Verification items for the finished model (mm, model axes). Round coordinates to 2 decimals unless told otherwise and drop trailing zeros. Write each loop counter-clockwise with the first axis right and the second up, starting at its lowest first coordinate (ties: lowest second). Pieces come first, ordered by that corner, then holes.
from build123d import *

# Parameters (mm, degrees)
SKETCH1_W           = 114.02881
SKETCH1_H           = 34
BOSS_EXTRUDE1_DEPTH = 10.01
SKETCH8_R           = 2.6
CUT_EXTRUDE3_DEPTH  = 120.410090068
SKETCH11_R          = 1.59
CUT_EXTRUDE6_DEPTH  = 120.410090068
SKETCH12_W          = 34
SKETCH12_H          = 10.01
BOSS_EXTRUDE2_DEPTH = 2.69
SKETCH14_W          = 34
SKETCH14_H          = 10.01
CUT_EXTRUDE7_DEPTH  = 2.69


with BuildPart() as part:
    # Sketch1 → Boss-Extrude1 (new body)
    with BuildSketch(Plane(origin=(0, 0, 0), x_dir=(1, 0, 0), z_dir=(0, 1, 0))):
        with Locations((57.014405, 17)):
            Rectangle(SKETCH1_W, SKETCH1_H)
    extrude(amount=BOSS_EXTRUDE1_DEPTH)

    # Sketch8 → Cut-Extrude3 (cut, through all)
    with BuildSketch(Plane(origin=(0, 0, -34), x_dir=(-1, 0, 0), z_dir=(0, 0, -1))):
        with Locations((-89.8, 5)):
            Circle(SKETCH8_R)
        with Locations((-29.8, 5)):
            Circle(SKETCH8_R)
    extrude(amount=-CUT_EXTRUDE3_DEPTH, mode=Mode.SUBTRACT)

    # Sketch11 → Cut-Extrude6 (cut, through all)
    with BuildSketch(Plane(origin=(0, 10.01, 0), x_dir=(1, 0, 0), z_dir=(0, 1, 0))):
        with Locations(Location((110.52881, 10.5, 0), (0, 0, 270))):
            Circle(SKETCH11_R)
        with Locations(Location((110.52881, 23.5, 0), (0, 0, 270))):
            Circle(SKETCH11_R)
        with Locations(Location((100.52881, 10.5, 0), (0, 0, 270))):
            Circle(SKETCH11_R)
        with Locations(Location((100.52881, 23.5, 0), (0, 0, 270))):
            Circle(SKETCH11_R)
    extrude(amount=-CUT_EXTRUDE6_DEPTH, mode=Mode.SUBTRACT)

    # Sketch12 → Boss-Extrude2 (add)
    with BuildSketch(Plane(origin=(114.02881, 0, 0), x_dir=(0, 0, -1), z_dir=(1, 0, 0))):
        with Locations((17, 5.005)):
            Rectangle(SKETCH12_W, SKETCH12_H)
    extrude(amount=BOSS_EXTRUDE2_DEPTH)

    # Sketch14 → Cut-Extrude7 (cut)
    with BuildSketch(Plane.ZY):
        with Locations((-17, 5.005)):
            Rectangle(SKETCH14_W, SKETCH14_H)
    extrude(amount=-CUT_EXTRUDE7_DEPTH, mode=Mode.SUBTRACT)


solid = part.part
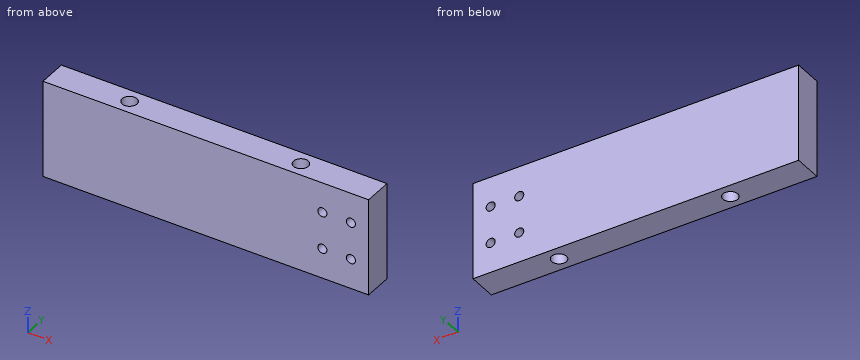
Q1. Material ranges on line 1 along X through (y, z) = (7.75, -11); line 2 along X through (y, z) = (4.25, -30); line 3 along X through (y, z) = (6.5, -23.5), recorded low to high.
Recorded:
line 1: x = 2.69 to 99.02, 102.04 to 109.02, 112.04 to 116.72
line 2: x = 2.69 to 27.31, 32.29 to 87.31, 92.29 to 116.72
line 3: x = 2.69 to 27.68, 31.92 to 87.68, 91.92 to 98.94, 102.12 to 108.94, 112.12 to 116.72
Q2. Sectioned sample at C-C (y = 5). Enter the section's corners in (x, z), plus the area to 3 significant figures.
Recorded:
outline: (2.69, -34) - (27.2, -34) - (27.2, 0) - (2.69, 0) - close; (32.4, -34) - (87.2, -34) - (87.2, 0) - (32.4, 0) - close; (92.4, -34) - (116.72, -34) - (116.72, 0) - (92.4, 0) - close; hole circle Ø3.18 at (100.53, -23.5); hole circle Ø3.18 at (100.53, -10.5); hole circle Ø3.18 at (110.53, -23.5); hole circle Ø3.18 at (110.53, -10.5)
area: 3,490 mm2
Q3. Depth check by flat-ended pin: P1, Ø4, axis at x = 89.8, y = 5, coming from the -Z side; P2, Ø6, axis at x = 38, y = 1, coming from the +Z side. Enter the tip coordinate at first touch or a pass-through.
Recorded:
P1: passes through
P2: stops at z = 0
Q4. Sectioned sample at A-A (z = -10.5). Enter the section's corners in (x, y), plus the area to 3 significant figures.
Recorded:
outline: (2.69, 0) - (98.94, 0) - (98.94, 10.01) - (2.69, 10.01) - close; (102.12, 0) - (108.94, 0) - (108.94, 10.01) - (102.12, 10.01) - close; (112.12, 0) - (116.72, 0) - (116.72, 10.01) - (112.12, 10.01) - close; hole circle Ø5.2 at (29.8, 5); hole circle Ø5.2 at (89.8, 5)
area: 1,040 mm2
Q5. Sectioned sample at B-B (x = 29.8). Enter the section's corners in (y, z).
Recorded:
outline: (0, -34) - (2.4, -34) - (2.4, 0) - (0, 0) - close; (7.6, -34) - (10.01, -34) - (10.01, 0) - (7.6, 0) - close
Q6. Sectioned sample at D-D (z = -6). Enter the section's corners in (x, y).
Recorded:
outline: (2.69, 0) - (116.72, 0) - (116.72, 10.01) - (2.69, 10.01) - close; hole circle Ø5.2 at (29.8, 5); hole circle Ø5.2 at (89.8, 5)
